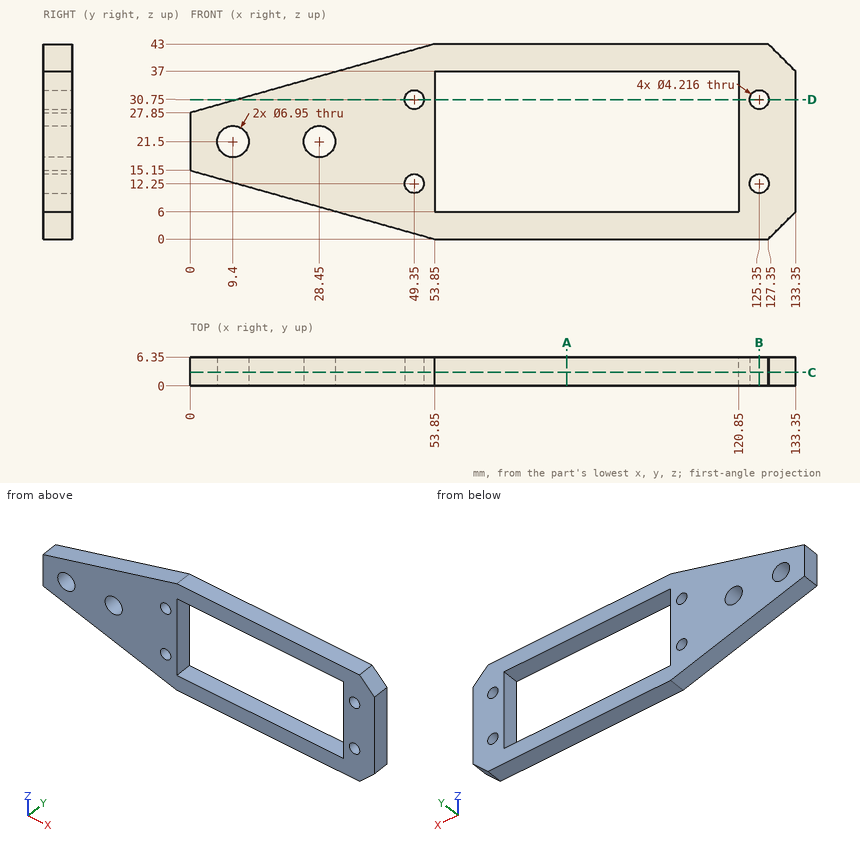
Can you work these out from the drawing? Everything is in mm from the part's minimum corner. Give positions to 0.01 mm unless a question says otherwise; leave off trailing zeros. Loops run counter-clockwise (first coordinate to the right, second up) from the corner with the lowest first, then second, coordinate; pieces in that order, holes last. Notation, with made-up numbers: M 37,-10.75 L 74,-10.75 A10 cw 74,-4.75 Z; hole C -23.5,-32.5 d2. An arc over 180 degrees is marked long. Use CSV: the item, a comma, the result in double quotes. Start each with the question number.
1. Imagine slicing it at C-C, the plane y = 3. Count the separate pieces of the cut face and the enclosed holes in it, plus the area to 3 significant figures.
2. For P1, Ø1.5, axis at x = 36.5, y = 3, coming from the -Z side, with a flat end and sliding along its axis, tell me the tip position at first contact or that it passes through.
3. Imagine slicing it at D-D, the plane z = 30.75. Write out the boundary of the cut face in (x, y), plus the area to 3 significant figures.
4. Imagine slicing it at A-A, the plane x = 83. Write out the boundary of the cut face in (y, z), plus the area to 3 significant figures.
5. If I drill on L1, parallel to X at y = 3, z = 15.5; L2, parallel to X at y = 3.75, z = 20.5; L3, parallel to Z at x = 99, y = 2.25, over which ranges is the centre line in solid material (lowest first)?
6. Imagine slicing it at B-B, the plane x = 125.35. Write out the boundary of the cut face in (y, z).
Response values:
1,separate pieces,"1"
1,enclosed holes,"7"
1,area,"2,670 mm^2"
2,P1,"z = 4.67"
3,outline,"M 10.31,0 L 47.24,0 L 47.24,6.35 L 10.31,6.35 Z; M 51.46,0 L 53.85,0 L 53.85,6.35 L 51.46,6.35 Z; M 120.85,0 L 123.24,0 L 123.24,6.35 L 120.85,6.35 Z; M 127.46,0 L 133.35,0 L 133.35,6.35 L 127.46,6.35 Z"
3,area,"302 mm^2"
4,outline,"M 0,0 L 6.35,0 L 6.35,6 L 0,6 Z; M 0,37 L 6.35,37 L 6.35,43 L 0,43 Z"
4,area,"76.2 mm^2"
5,L1,"0 to 53.85, 120.85 to 133.35"
5,L2,"0 to 6.07, 12.73 to 25.12, 31.78 to 53.85, 120.85 to 133.35"
5,L3,"0 to 6, 37 to 43"
6,outline,"M 0,0 L 6.35,0 L 6.35,10.14 L 0,10.14 Z; M 0,14.36 L 6.35,14.36 L 6.35,28.64 L 0,28.64 Z; M 0,32.86 L 6.35,32.86 L 6.35,43 L 0,43 Z"
